The model under review builds one solid part; all positions refer to its coordinate system, in mm. Coordinates: 2 decimals unless noted, no trailing zeros. Loops run counter-clockwise (first coordinate to the right, second up) from the corner with the lowest first, then second, coordinate; pieces in that order, holes last. Notation, with made-up numbers: (49, 24.25) - (78, 24.25) arc R37 cw to (78, 63.25) - close; hole circle Ø6 at (29, -38). An arc over 180 degrees is marked (long way). Use a Markdown table: item, result. Add a question column.
1) Add section D-D, the plane x = 3.5. Give the boundary of the cut face in (y, z), and give its area (3 significant figures).
2) Add section B-B, the plane z = 3.25. Give the boundary of the cut face in (x, y), and give its area (3 significant figures).
3) Add section C-C, the plane y = 0.15. Give the boundary of the cut face in (x, z), and give its area (3 significant figures).
4) To check wall thickness, follow L1, parallel to X at y = 0.2, z = 0; L2, parallel to X at y = 0.2, z = 2.75. State the ranges of each line that lie inside material, in increasing order. Write a range as [from, to].
5) Add section A-A, the plane x = 0. Give the boundary of the cut face in (y, z).
```python
from build123d import *

# Parameters (mm, degrees)
SKETCH1_W           = 21
SKETCH1_H           = 21
BOSS_EXTRUDE1_DEPTH = 0.58
SKETCH2_W           = 10.5
SKETCH2_H           = 10.5
CUT_EXTRUDE1_DEPTH  = 15.860565265
FILLET1_R           = 2
SKETCH5_R           = 1.1
CUT_EXTRUDE5_DEPTH  = 15.860565265
FILLET2_R           = 0.4


with BuildPart() as part:
    # Sketch1 → Boss-Extrude1 (new body)
    with BuildSketch(Plane(origin=(0, 0, 0), x_dir=(1, 0, 0), z_dir=(0, 1, 0))):
        Rectangle(SKETCH1_W, SKETCH1_H)
    extrude(amount=BOSS_EXTRUDE1_DEPTH)

    # Sketch2 → Cut-Extrude1 (cut, through all)
    with BuildSketch(Plane(origin=(0, 0.58, 0), x_dir=(1, 0, 0), z_dir=(0, 1, 0))):
        Rectangle(SKETCH2_W, SKETCH2_H)
    extrude(amount=-CUT_EXTRUDE1_DEPTH, mode=Mode.SUBTRACT)

    # Fillet1
    fillet1_edges = [part.edges().sort_by_distance(p)[0] for p in [
        (10.5, 0.29, 10.5),
        (-10.5, 0.29, 10.5),
        (-10.5, 0.29, -10.5),
        (10.5, 0.29, -10.5),
    ]]
    fillet(fillet1_edges, radius=FILLET1_R)

    # Sketch5 → Cut-Extrude5 (cut, through all)
    with BuildSketch(Plane(origin=(0, 0.58, 0), x_dir=(1, 0, 0), z_dir=(0, 1, 0))):
        with Locations(Location((0, 8.3, 0), (0, 0, 270))):
            Circle(SKETCH5_R)
        with Locations(Location((8.3, 0, 0), (0, 0, 270))):
            Circle(SKETCH5_R)
        with Locations(Location((0, -8.3, 0), (0, 0, 270))):
            Circle(SKETCH5_R)
        with Locations(Location((-8.3, 0, 0), (0, 0, 270))):
            Circle(SKETCH5_R)
    extrude(amount=-CUT_EXTRUDE5_DEPTH, mode=Mode.SUBTRACT)

    # Fillet2
    fillet2_edges = [part.edges().sort_by_distance(p)[0] for p in [
        (5.25, 0.29, -5.25),
        (5.25, 0.29, 5.25),
        (-5.25, 0.29, 5.25),
        (-5.25, 0.29, -5.25),
    ]]
    fillet(fillet2_edges, radius=FILLET2_R)


solid = part.part
```
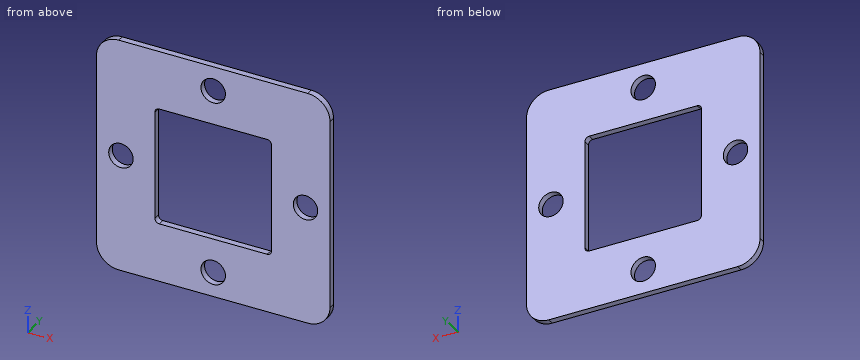
From the geometry:
| question | item | result |
|---|---|---|
| 1 | outline | (0, -10.5) - (0.58, -10.5) - (0.58, -5.25) - (0, -5.25) - close; (0, 5.25) - (0.58, 5.25) - (0.58, 10.5) - (0, 10.5) - close |
| 1 | area | 6.09 mm^2 |
| 2 | outline | (-10.5, 0) - (-5.25, 0) - (-5.25, 0.58) - (-10.5, 0.58) - close; (5.25, 0) - (10.5, 0) - (10.5, 0.58) - (5.25, 0.58) - close |
| 2 | area | 6.09 mm^2 |
| 3 | outline | (-10.5, -8.5) arc R2 ccw to (-8.5, -10.5) - (8.5, -10.5) arc R2 ccw to (10.5, -8.5) - (10.5, 8.5) arc R2 ccw to (8.5, 10.5) - (-8.5, 10.5) arc R2 ccw to (-10.5, 8.5) - close; hole circle Ø2.2 at (-8.3, 0); hole (-5.25, -4.85) arc R0.4 ccw to (-4.85, -5.25) - (4.85, -5.25) arc R0.4 ccw to (5.25, -4.85) - (5.25, 4.85) arc R0.4 ccw to (4.85, 5.25) - (-4.85, 5.25) arc R0.4 ccw to (-5.25, 4.85) - close; hole circle Ø2.2 at (0, -8.3); hole circle Ø2.2 at (0, 8.3); hole circle Ø2.2 at (8.3, 0) |
| 3 | area | 312 mm^2 |
| 4 | L1 | x = [-10.5, -9.4], [-7.2, -5.25], [5.25, 7.2], [9.4, 10.5] |
| 4 | L2 | x = [-10.5, -5.25], [5.25, 10.5] |
| 5 | outline | (0, -10.5) - (0.58, -10.5) - (0.58, -9.4) - (0, -9.4) - close; (0, -7.2) - (0.58, -7.2) - (0.58, -5.25) - (0, -5.25) - close; (0, 5.25) - (0.58, 5.25) - (0.58, 7.2) - (0, 7.2) - close; (0, 9.4) - (0.58, 9.4) - (0.58, 10.5) - (0, 10.5) - close |
